Print and shaded views of the part. All mm, measured from the part's lowest x, y and z. Coordinates: 2 decimals unless noted, no trailing zeros. Loops run counter-clockwise (first coordinate to the right, second up) from the corner with the lowest first, then second, coordinate; pieces in that order, holes last. Notation, with made-up numbers: (36.5, 69.5) -> (49.5, 69.5) arc R19 cw to (49.5, 99.5) -> close; hole circle Ø2 at (-28, 63.25). An arc over 180 degrees is marked (long way). One line per item, written item: value. Start each with the question number.
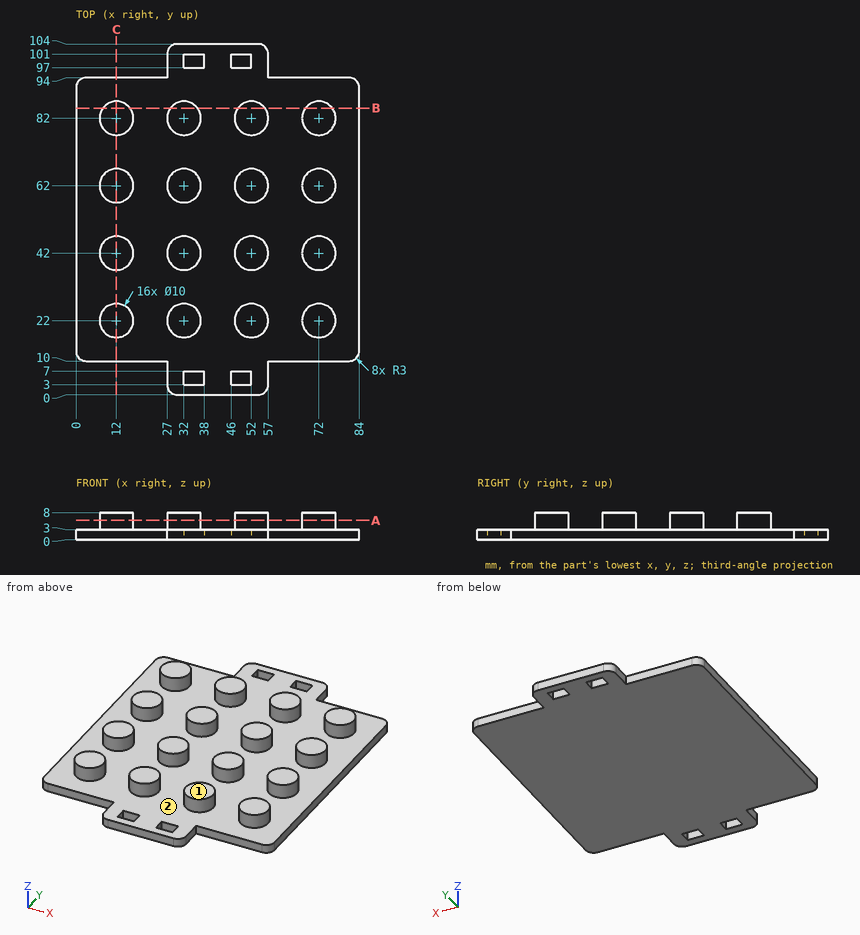
1) Probe line 1 (X direction, y = 61, z = 4); line 2 (X direction, y = 21.5, z = 7.75); line 3 (Z direction, x = 64, y = 72.5). List the from-to ranges inside material, lowest first. Write a range as from..to.
2) Slice it at A-A (z = 5.75). State how many separate pieces and enclosed holes the cut face has, then the cut area to 3 significant figures.
3) Slice it at B-B (y = 85). Give the cut face in (x, z).
4) Pin check, flat tips, straight feed: pin 1 Ø1.5 at (y, z) = (96, 1) entering from -X; pin 2 Ø4 at (x, y) = (69.5, 32.5) entering from +Z; pin 3 Ø1.5 at (y, z) = (5.5, 2) entering from +X; pin 4 Ø0.9 at (x, z) = (49.5, 1) entering from -Y. Stop position of each tip, or through.
5) Pull direction X, two halves, no side cores. Call the marked faces 1 and 2: +X half, -X half, draft (parallel to the pull), parting line (faces both ways), or undercut.
6) Slice it at C-C (x = 12). Give the cut face in (y, z), then the cut area to 3 significant figures.
Check sheet entries:
1. line 1: x = 7.1..16.9, 27.1..36.9, 47.1..56.9, 67.1..76.9
1. line 2: x = 7.03..16.97, 27.03..36.97, 47.03..56.97, 67.03..76.97
1. line 3: z = 0..3
2. separate pieces: 16
2. enclosed holes: 0
2. area: 1,260 mm^2
3. outline: (0, 0) -> (84, 0) -> (84, 3) -> (76, 3) -> (76, 8) -> (68, 8) -> (68, 3) -> (56, 3) -> (56, 8) -> (48, 8) -> (48, 3) -> (36, 3) -> (36, 8) -> (28, 8) -> (28, 3) -> (16, 3) -> (16, 8) -> (8, 8) -> (8, 3) -> (0, 3) -> close
4. pin 1: stops at x = 27
4. pin 2: stops at z = 3
4. pin 3: stops at x = 57
4. pin 4: stops at y = 0
5. face 1: draft
5. face 2: undercut
6. outline: (10, 0) -> (94, 0) -> (94, 3) -> (87, 3) -> (87, 8) -> (77, 8) -> (77, 3) -> (67, 3) -> (67, 8) -> (57, 8) -> (57, 3) -> (47, 3) -> (47, 8) -> (37, 8) -> (37, 3) -> (27, 3) -> (27, 8) -> (17, 8) -> (17, 3) -> (10, 3) -> close
6. area: 452 mm^2
